Verification items for the finished model (mm, model axes). A direction names the side the tool comes from. Round coordinates to 2 decimals unless told otherwise and drop trailing zeros. Write each loop counter-clockwise with the first axis right and the second up, starting at its lowest first coordinate (ties: lowest second). Pieces come first, ordered by that corner, then holes. Notation, with made-up numbers: M 59,38.5 L 98,38.5 A18 ccw 98,52.5 Z; hole C 21,27 d4. An arc over 180 degrees is marked long. Answer in a Markdown table with one row per item. Add a question column.
1. Material ranges on probe 1 along Y at (x, z) = (44, 4.35); probe 2 along Y at (x, z) = (16, 4); probe 3 along Y at (x, z) = (38.5, 2.25), recorded low to high.
2. Go/stop test with flat-tipped pins: pin 1 Ø6 at (x, y) = (-6.5, -13) entering from -Z; pin 2 Ø4 at (x, y) = (-44, -24) entering from -Z; pin 3 Ø5.5 at (x, y) = (44, -24) entering from +Z; pin 4 Ø11.5 at (x, y) = (-37, -35) entering from -Z. Record where each tip stops, or that it passes through.
3. Set-up check for faces 1 (the flat face through (44, -26, 8)), 2 (the flat face through (-49.1, -1, 10)), 3 (the flat face through (17, -28.3, 4)), 4 (the cylindrical face through (41, -24, 2)): record each of +Z, -Z, +X, -X, +Y, -Y from which the full face is reachable in a straight line by a thin tool's end or side.
4. Sectioned sample at B-B on y = 16.5. Record the cut outline in (x, z).
5. Sectioned sample at A-A on x = -4. Record the cut outline in (y, z).
6. Draft check along Y on faces 5 (the cylindrical face through (-43.1, -22.5, 5.7)), 6 (the flat face through (-1, -19, 0)). Enter one of: pulls with the +Y half, pulls with the -Y half, needs draft (parallel to the pull), parting line crosses it, or undercut.
7. Sectioned sample at C-C on x = -18.5. Record the cut outline in (y, z), plus the area to 3 significant figures.
8. Sectioned sample at D-D on y = -24. Count the separate pieces of the cut face and the enclosed holes in it, plus the area to 3 significant figures.
```python
from build123d import *

# Parameters (mm, degrees)
SKETCH_W      = 98.2
SKETCH_H      = 92.2
SKETCH_R      = 5
SKETCH_R_2    = 3.2
SKETCH_R_3    = 1.4
SKETCH_R_4    = 2.2
SKETCH_R_5    = 3
SKETCH_W_2    = 79
SKETCH_H_2    = 52
SKETCH_W_3    = 23
SKETCH_H_3    = 10.5
PAD_DEPTH     = 1.8
SKETCH001_W   = 98.2
SKETCH001_H   = 92.2
SKETCH001_W_2 = 95
SKETCH001_H_2 = 89
PAD001_DEPTH  = 15.7
SKETCH002_R   = 4.2
SKETCH002_R_2 = 3
PAD002_DEPTH  = 1.6
SKETCH026_R   = 4.2
SKETCH026_R_2 = 1.75
PAD013_DEPTH  = 4.6
SKETCH027_W   = 24.64
SKETCH027_H   = 12.14
SKETCH027_W_2 = 23
SKETCH027_H_2 = 10.5
PAD014_DEPTH  = 6.2
SKETCH003_W   = 27
SKETCH003_H   = 4
POCKET_DEPTH  = 1.6
FILLET_R      = 1.799


with BuildPart() as part:
    # Sketch → Pad (new body)
    with BuildSketch(Plane.XY):
        Rectangle(SKETCH_W, SKETCH_H)
        with Locations((-37, -35)):
            Circle(SKETCH_R, mode=Mode.SUBTRACT)
        with Locations((-4, -35)):
            Circle(SKETCH_R_2, mode=Mode.SUBTRACT)
        with Locations((-23.1, -35)):
            Circle(SKETCH_R_3, mode=Mode.SUBTRACT)
        with Locations((-18.5, -30.4)):
            Circle(SKETCH_R_3, mode=Mode.SUBTRACT)
        with Locations((-13.9, -35)):
            Circle(SKETCH_R_3, mode=Mode.SUBTRACT)
        with Locations((-18.5, -39.6)):
            Circle(SKETCH_R_3, mode=Mode.SUBTRACT)
        with Locations((-18.5, -35)):
            Circle(SKETCH_R_4, mode=Mode.SUBTRACT)
        with Locations((-21.752691, -31.747309)):
            Circle(SKETCH_R_3, mode=Mode.SUBTRACT)
        with Locations((-15.247309, -31.747309)):
            Circle(SKETCH_R_3, mode=Mode.SUBTRACT)
        with Locations((-15.247309, -38.252691)):
            Circle(SKETCH_R_3, mode=Mode.SUBTRACT)
        with Locations((-21.752691, -38.252691)):
            Circle(SKETCH_R_3, mode=Mode.SUBTRACT)
        with Locations((38.5, -31.5)):
            Circle(SKETCH_R_2, mode=Mode.SUBTRACT)
        with Locations((-44, 41.5)):
            Circle(SKETCH_R_5, mode=Mode.SUBTRACT)
        with Locations((44, 41.5)):
            Circle(SKETCH_R_5, mode=Mode.SUBTRACT)
        with Locations((-44, -24)):
            Circle(SKETCH_R_5, mode=Mode.SUBTRACT)
        with Locations((44, -24)):
            Circle(SKETCH_R_5, mode=Mode.SUBTRACT)
        with Locations((0, 9)):
            Rectangle(SKETCH_W_2, SKETCH_H_2, mode=Mode.SUBTRACT)
        with Locations((17.25, -33.55)):
            Rectangle(SKETCH_W_3, SKETCH_H_3, mode=Mode.SUBTRACT)
    extrude(amount=PAD_DEPTH)

    # Sketch001 → Pad001 (join)
    with BuildSketch(Plane.XY.offset(1.8)):
        Rectangle(SKETCH001_W, SKETCH001_H)
        Rectangle(SKETCH001_W_2, SKETCH001_H_2, mode=Mode.SUBTRACT)
    extrude(amount=PAD001_DEPTH)

    # Sketch002 → Pad002 (join)
    with BuildSketch(Plane.XY.offset(1.8)):
        with Locations((-44, 41.5)):
            Circle(SKETCH002_R)
        with Locations((-44, 41.5)):
            Circle(SKETCH002_R_2, mode=Mode.SUBTRACT)
        with Locations((44, 41.5)):
            Circle(SKETCH002_R)
        with Locations((44, 41.5)):
            Circle(SKETCH002_R_2, mode=Mode.SUBTRACT)
        with Locations((44, -24)):
            Circle(SKETCH002_R)
        with Locations((44, -24)):
            Circle(SKETCH002_R_2, mode=Mode.SUBTRACT)
        with Locations((-44, -24)):
            Circle(SKETCH002_R)
        with Locations((-44, -24)):
            Circle(SKETCH002_R_2, mode=Mode.SUBTRACT)
    extrude(amount=PAD002_DEPTH)

    # Sketch026 → Pad013 (join)
    with BuildSketch(Plane.XY.offset(3.4)):
        with Locations((-44, 41.5)):
            Circle(SKETCH026_R)
        with Locations((-44, 41.5)):
            Circle(SKETCH026_R_2, mode=Mode.SUBTRACT)
        with Locations((44, 41.5)):
            Circle(SKETCH026_R)
        with Locations((44, 41.5)):
            Circle(SKETCH026_R_2, mode=Mode.SUBTRACT)
        with Locations((44, -24)):
            Circle(SKETCH026_R)
        with Locations((44, -24)):
            Circle(SKETCH026_R_2, mode=Mode.SUBTRACT)
        with Locations((-44, -24)):
            Circle(SKETCH026_R)
        with Locations((-44, -24)):
            Circle(SKETCH026_R_2, mode=Mode.SUBTRACT)
    extrude(amount=PAD013_DEPTH)

    # Sketch027 → Pad014 (join)
    with BuildSketch(Plane.XY.offset(1.8)):
        with Locations((17.25, -33.55)):
            Rectangle(SKETCH027_W, SKETCH027_H)
        with Locations((17.25, -33.55)):
            Rectangle(SKETCH027_W_2, SKETCH027_H_2, mode=Mode.SUBTRACT)
    extrude(amount=PAD014_DEPTH)

    # Sketch003 → Pocket (cut)
    with BuildSketch(Plane.YZ.offset(49.1)):
        with Locations((8.5, 15.5)):
            Rectangle(SKETCH003_W, SKETCH003_H)
    extrude(amount=-POCKET_DEPTH, mode=Mode.SUBTRACT)

    # Fillet
    fillet_edges = [part.edges().sort_by_distance(p)[0] for p in [
        (-49.1, -46.1, 8.75),
        (0, -46.1, 0),
        (-49.1, 0, 0),
        (-49.1, 46.1, 8.75),
        (49.1, -46.1, 8.75),
        (49.1, 0, 0),
        (0, 46.1, 0),
        (49.1, 46.1, 8.75),
    ]]
    fillet(fillet_edges, radius=FILLET_R)


solid = part.part
```
Geometry check:
| question | item | result |
|---|---|---|
| 1 | probe 1 | y = -46.1 to -44.5, -28.2 to -25.75, -22.25 to -19.8, 37.3 to 39.75, 43.25 to 46.1 |
| 1 | probe 2 | y = -46.1 to -44.5, -39.62 to -38.8, -28.3 to -27.48, 44.5 to 46.1 |
| 1 | probe 3 | y = -46.1 to -44.5, 44.5 to 46.1 |
| 2 | pin 1 | passes through |
| 2 | pin 2 | stops at z = 3.4 |
| 2 | pin 3 | stops at z = 8 |
| 2 | pin 4 | stops at z = 0 |
| 3 | face 1 | +Z |
| 3 | face 2 | +Z, -Z, -X, +Y, -Y |
| 3 | face 3 | +Z, -Z |
| 3 | face 4 | -Z |
| 4 | outline | M -49.1,1.8 A1.8 ccw -47.3,0 L -39.5,0 L -39.5,1.8 L -47.5,1.8 L -47.5,17.5 L -49.1,17.5 Z; M 39.5,0 L 47.3,0 A1.8 ccw 49.1,1.8 L 49.1,13.5 L 47.5,13.5 L 47.5,1.8 L 39.5,1.8 Z |
| 5 | outline | M -46.1,1.8 A1.8 ccw -44.3,0 L -38.2,0 L -38.2,1.8 L -44.5,1.8 L -44.5,17.5 L -46.1,17.5 Z; M -31.8,0 L -17,0 L -17,1.8 L -31.8,1.8 Z; M 35,0 L 44.3,0 A1.8 ccw 46.1,1.8 L 46.1,17.5 L 44.5,17.5 L 44.5,1.8 L 35,1.8 Z |
| 6 | face 5 | undercut |
| 6 | face 6 | needs draft |
| 7 | outline | M -46.1,1.8 A1.8 ccw -44.3,0 L -41,0 L -41,1.8 L -44.5,1.8 L -44.5,17.5 L -46.1,17.5 Z; M -38.2,0 L -37.2,0 L -37.2,1.8 L -38.2,1.8 Z; M -32.8,0 L -31.8,0 L -31.8,1.8 L -32.8,1.8 Z; M -29,0 L -17,0 L -17,1.8 L -29,1.8 Z; M 35,0 L 44.3,0 A1.8 ccw 46.1,1.8 L 46.1,17.5 L 44.5,17.5 L 44.5,1.8 L 35,1.8 Z |
| 7 | area | 103 mm2 |
| 8 | separate pieces | 3 |
| 8 | enclosed holes | 0 |
| 8 | area | 248 mm2 |
